```python
from build123d import *

# Parameters (mm, degrees)
SKETCH1_W           = 25
SKETCH1_H           = 20.5
BOSS_EXTRUDE1_DEPTH = 48.5
SKETCH2_R           = 4.25
CUT_EXTRUDE1_DEPTH  = 3.5
SKETCH3_R           = 2.5
CUT_EXTRUDE2_DEPTH  = 17
SKETCH4_R           = 6.5
CUT_EXTRUDE3_DEPTH  = 25
SKETCH5_R           = 2.5
CUT_EXTRUDE4_DEPTH  = 10


with BuildPart() as part:
    # Sketch1 → Boss-Extrude1 (new body)
    with BuildSketch(Plane.XY):
        with Locations((11.55511811, 8.921259843)):
            Rectangle(SKETCH1_W, SKETCH1_H)
    extrude(amount=BOSS_EXTRUDE1_DEPTH)

    # Sketch2 → Cut-Extrude1 (cut)
    with BuildSketch(Plane(origin=(0, 19.171259843, 0), x_dir=(1, 0, 0), z_dir=(0, 1, 0))):
        with Locations((11.55511811, -39.5)):
            Circle(SKETCH2_R)
        with Locations((11.55511811, -9)):
            Circle(SKETCH2_R)
    extrude(amount=-CUT_EXTRUDE1_DEPTH, mode=Mode.SUBTRACT)

    # Sketch3 → Cut-Extrude2 (cut)
    with BuildSketch(Plane(origin=(0, 15.671259843, 0), x_dir=(1, 0, 0), z_dir=(0, 1, 0))):
        with Locations((11.55511811, -39.5)):
            Circle(SKETCH3_R)
        with Locations((11.55511811, -9)):
            Circle(SKETCH3_R)
    extrude(amount=-CUT_EXTRUDE2_DEPTH, mode=Mode.SUBTRACT)

    # Sketch4 → Cut-Extrude3 (cut)
    with BuildSketch(Plane(origin=(24.05511811, 0, 0), x_dir=(0, 0, -1), z_dir=(1, 0, 0))):
        with Locations((-24.25, 8.921259843)):
            Circle(SKETCH4_R)
    extrude(amount=-CUT_EXTRUDE3_DEPTH, mode=Mode.SUBTRACT)

    # Sketch5 → Cut-Extrude4 (cut)
    with BuildSketch(Plane(origin=(24.05511811, 0, 0), x_dir=(0, 0, -1), z_dir=(1, 0, 0))):
        with Locations((-13, 8.921259843)):
            Circle(SKETCH5_R)
        with Locations((-35.5, 8.921259843)):
            Circle(SKETCH5_R)
    extrude(amount=-CUT_EXTRUDE4_DEPTH, mode=Mode.SUBTRACT)


solid = part.part
```
Geometry check sheet. Reference: the model listing, model coordinates, mm. A direction names the side the tool comes from. Give positions to 0.01 mm unless a question says otherwise; leave off trailing zeros. Write each loop counter-clockwise with the first axis right and the second up, starting at its lowest first coordinate (ties: lowest second). Pieces come first, ordered by that corner, then holes. Notation, with made-up numbers: (-9, 89) - (46, 89) arc R4 cw to (46, 94) - close; hole circle Ø10 at (9.25, 62.5). An arc over 180 degrees is marked (long way). Use a Markdown table: item, result.
Q1. Section check C-C, the plane y = 0.5. Enter the section's corners in (x, z), then the cut area to 3 significant figures.
Computed:
| item | result |
|---|---|
| outline | (-0.94, 0) - (24.06, 0) - (24.06, 48.5) - (-0.94, 48.5) - close; hole circle Ø5 at (11.56, 9); hole circle Ø5 at (11.56, 39.5) |
| area | 1,170 mm² |
Q2. Thickness scan on L1, parallel to X at y = 7.25, z = 39.5; L2, parallel to Z at x = 22.75, y = 8; L3, parallel to Y at x = 9, z = 24. Record the ranges inside material, lowest first. Write a range as [from, to].
Computed:
| item | result |
|---|---|
| L1 | x = [-0.94, 9.06], [14.06, 24.06] |
| L2 | z = [0, 10.68], [15.32, 17.82], [30.68, 33.18], [37.82, 48.5] |
| L3 | y = [-1.33, 2.43], [15.42, 19.17] |
Q3. Section check D-D, the plane z = 24.25. Enter the section's corners in (x, y).
Computed:
| item | result |
|---|---|
| outline | (-0.94, -1.33) - (24.06, -1.33) - (24.06, 2.42) - (-0.94, 2.42) - close; (-0.94, 15.42) - (24.06, 15.42) - (24.06, 19.17) - (-0.94, 19.17) - close |
Q4. Section check A-A, the plane y = 8. Enter the section's corners in (x, z), then the cut area to 3 significant figures.
Computed:
| item | result |
|---|---|
| outline | (-0.94, 0) - (24.06, 0) - (24.06, 10.68) - (14.06, 10.68) - (14.06, 15.32) - (24.06, 15.32) - (24.06, 17.82) - (-0.94, 17.82) - close; (-0.94, 30.68) - (24.06, 30.68) - (24.06, 33.18) - (14.06, 33.18) - (14.06, 37.82) - (24.06, 37.82) - (24.06, 48.5) - (-0.94, 48.5) - close; hole circle Ø5 at (11.56, 9); hole circle Ø5 at (11.56, 39.5) |
| area | 759 mm² |
Q5. Go/stop test with flat-tipped pins: P1, Ø2.5, axis at x = 13, z = 38.5, coming from the +Y side; P2, Ø2.5, axis at y = 8.5, z = 14, coming from the +X side. Record where each tip stops, or that it passes through.
Computed:
| item | result |
|---|---|
| P1 | stops at y = 15.67 |
| P2 | stops at x = 14.06 |
Q6. Set-up check for faces 1 (the face through (19.125, 7.964, 33.191)), 2 (the face through (11.01, 7.29, 11.44)), 3 (the face through (11, 15.671, 12)): record each of +Z, -Z, +X, -X, +Y, -Y from which the full face is reachable in a straight line by a thin tool's end or side.
Computed:
| item | result |
|---|---|
| face 1 | +X |
| face 2 | +Y, -Y |
| face 3 | +Y |
Q7. Draft check along Y on faces 4 (the face through (11.73, 9.207, 30.744)), 5 (the face through (24.055, 2, 24)), 6 (the face through (11, -1.329, 24)). Enter one of: pulls with the +Y half, pulls with the -Y half, needs draft (parallel to the pull), parting line crosses it, or undercut.
Computed:
| item | result |
|---|---|
| face 4 | undercut |
| face 5 | needs draft |
| face 6 | pulls with the -Y half |
Q8. Section check B-B, the plane z = 39.5. Enter the section's corners in (x, y).
Computed:
| item | result |
|---|---|
| outline | (-0.94, -1.33) - (9.06, -1.33) - (9.06, 15.67) - (7.31, 15.67) - (7.31, 19.17) - (-0.94, 19.17) - close; (14.06, -1.33) - (24.06, -1.33) - (24.06, 19.17) - (15.81, 19.17) - (15.81, 15.67) - (14.06, 15.67) - close |
